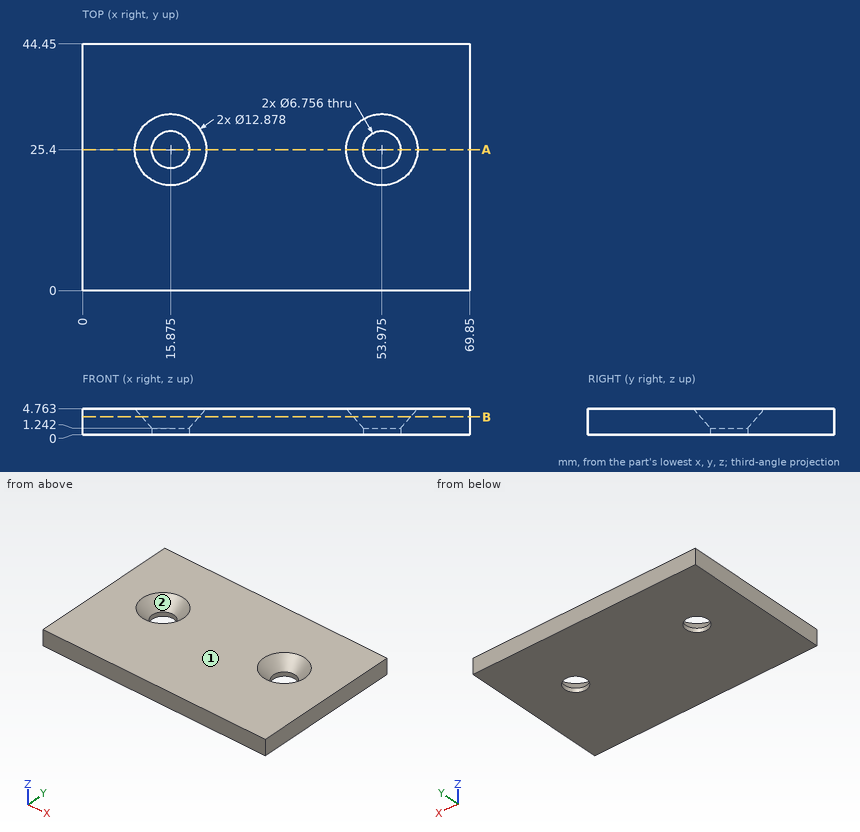
Part print with two shaded views. Sizes in mm from the minimum x, y, z corner. Coordinates: 2 decimals unless noted, no trailing zeros. Order: outer loops, then holes, each group sorted by start corner. A loop starts at its lowest first (then second) coordinate and runs counter-clockwise, first axis right, second up. Notation, with made-up numbers: M -39.5,8 L -11.5,8 A3 ccw -11.5,12 Z; hole C 39.5,-23.5 d3. An arc over 180 degrees is marked long. Use a Markdown table: item, result.
(1) Cut at B-B on z = 3.25. State how many separate pieces and enclosed holes the cut face has, then the cut area to 3 significant figures.
A:
| item | result |
|---|---|
| separate pieces | 1 |
| enclosed holes | 2 |
| area | 2,940 mm^2 |
(2) Probe L1, parallel to X at y = 25.4, z = 0.8; L2, parallel to Y at x = 16.5, z = 4; L3, parallel to Z at x = 58, y = 25.5 (1 decimal). List the from-to ranges inside material, lowest first.
A:
| item | result |
|---|---|
| L1 | x = 0 to 12.5, 19.25 to 50.6, 57.35 to 69.85 |
| L2 | y = 0 to 19.66, 31.14 to 44.45 |
| L3 | z = 0 to 2 |
(3) Pull direction Y, two halves, no side cores. Call the marked faces 1 and 2: released by +Y, released by -Y, zero draft, split by the parting line, or undercut.
A:
| item | result |
|---|---|
| face 1 | zero draft |
| face 2 | undercut |
(4) Cut at A-A on y = 25.4. Write the cut outline in (x, z), then the cut area to 3 significant figures.
A:
| item | result |
|---|---|
| outline | M 0,0 L 12.5,0 L 12.5,1.24 L 9.44,4.76 L 0,4.76 Z; M 19.25,0 L 50.6,0 L 50.6,1.24 L 47.54,4.76 L 22.31,4.76 L 19.25,1.24 Z; M 57.35,0 L 69.85,0 L 69.85,4.76 L 60.41,4.76 L 57.35,1.24 Z |
| area | 247 mm^2 |
